```python
from build123d import *

# Parameters (mm, degrees)
F1_DEPTH       = 25.4
F3_D           = 7.874
F3_CBORE_D     = 12.7
F3_CBORE_DEPTH = 6.096
F5_DEPTH       = 12.7
F6_DEPTH       = 105.8292752574
F7_W           = 19.304
F7_H           = 6.096
F8_DEPTH       = 66.549


with BuildPart() as f1:
    # F0 (on Front) → F1 (new body, symmetric)
    with BuildSketch(Plane.XZ):
        Polygon((-85.852, 0), (0, 0), (45.8512699094, -45.8512699094), (54.8315260304, -36.8710137883), (5.2605122421, 12.7), (-85.852, 12.7), align=None)
    extrude(amount=F1_DEPTH, both=True)

    # F3 (through all)
    with Locations(Plane(origin=(0, 0, 0), x_dir=(1, 0, 0), z_dir=(0, 0, -1))):
        with Locations((-70.104, 12.7), (-16.256, 12.7), (-16.256, -12.7), (-70.104, -12.7)):
            CounterBoreHole(F3_D / 2, F3_CBORE_D / 2, F3_CBORE_DEPTH)

    # F4 (on face) → F5 (join)
    with BuildSketch(Plane(origin=(8.9802561211, 0, 8.9802561211), x_dir=(0.7071067812, 0, -0.7071067812), z_dir=(0.7071067812, 0, 0.7071067812))):
        with BuildLine():
            Line((10.9954877579, -25.4), (58.4765061126, -25.4))
            ThreePointArc((58.4765061126, -25.4), (64.8434877579, 0), (58.4765061126, 25.4))
            Line((58.4765061126, 25.4), (10.9954877579, 25.4))
            Line((10.9954877579, 25.4), (10.9954877579, -25.4))
        make_face()
    extrude(amount=F5_DEPTH)

    # F6 (cut, through all): faces of the model
    f6_faces = [f1.faces().sort_by_distance(p)[0] for p in [
        (53.495770348, -19.1275210106, -35.5352581058),
        (53.495770348, 19.1275210106, -35.5352581058),
    ]]
    extrude(f6_faces, amount=-F6_DEPTH, mode=Mode.SUBTRACT)

    # F7 (on face) → F8 (cut, through all)
    with BuildSketch(Plane(origin=(7.774983956, 0, -7.774983956), x_dir=(0, -1, 0), z_dir=(-0.7071067812, 0, 0.7071067812))):
        Polygon((-15.748, 19.304), (-15.748, 12.7), (15.748, 12.7), (15.748, 19.304), (9.652, 19.304), (-9.652, 19.304), align=None)
        with Locations((0, 22.352)):
            Rectangle(F7_W, F7_H)
    extrude(amount=-F8_DEPTH, mode=Mode.SUBTRACT)


solid = f1.part
```
For this review, take the finished solid that the model builds, in its own axes (mm). A direction names the side the tool comes from. Round coordinates to 2 decimals unless told otherwise and drop trailing zeros. Write each loop counter-clockwise with the first axis right and the second up, starting at its lowest first coordinate (ties: lowest second). Pieces come first, ordered by that corner, then holes. Notation, with made-up numbers: (-28, -27.75) - (-9, -27.75) arc R13 cw to (-9, -21.75) - close; hole circle Ø8 at (15.25, 73.25). An arc over 180 degrees is marked (long way). Use CSV: the item, a comma, the result in double quotes.
1) Add section D-D on z = -13.5. Write out the cut boundary in (x, y).
Conclusion:
outline,"(13.5, -25.4) - (49.42, -25.4) - (49.42, -9.65) - (40.8, -9.65) - (40.8, -15.75) - (31.46, -15.75) - (31.46, 15.75) - (40.8, 15.75) - (40.8, 9.65) - (49.42, 9.65) - (49.42, 25.4) - (13.5, 25.4) - close"
2) Add section A-A on y = 12.7. Write out the cut boundary in (x, z) (1 decimal), and give its area (3 significant figures).
Conclusion:
outline,"(-85.9, 0) - (-76.5, 0) - (-76.5, 6.1) - (-74, 6.1) - (-74, 12.7) - (-85.9, 12.7) - close; (-66.2, 6.1) - (-63.8, 6.1) - (-63.8, 0) - (-22.6, 0) - (-22.6, 6.1) - (-20.2, 6.1) - (-20.2, 12.7) - (-66.2, 12.7) - close; (-12.3, 6.1) - (-9.9, 6.1) - (-9.9, 0) - (0, 0) - (44.8, -44.8) - (53.8, -35.8) - (5.3, 12.7) - (-12.3, 12.7) - close; (21.4, 5.9) - (58.4, -31.1) - (62.7, -26.8) - (25.7, 10.2) - close"
area,"2,020 mm^2"
3) The part is to be moulded in two halves that separate along Y. For faces 1 (the cylindrical face through (53, -0.4, -38.7)), 2 (the flat face through (-67, -16, 6.096)), 3 (the cylindrical face through (-19.89, 14.21, 9.44)), 4 (the flat face through (22.18, -19.17, 6.63)), say which applies: pulls with the +Y half, pulls with the -Y half, needs draft (parallel to the pull), parting line crosses it, or undercut.
Conclusion:
face 1,"parting line crosses it"
face 2,"undercut"
face 3,"undercut"
face 4,"needs draft"
4) For faces 5 (the flat face through (23, 0, -23)), 6 (the cylindrical face through (-17.083, -18.996, 3.005)), 7 (the flat face through (42, 9.652, -10)), 8 (the cylindrical face through (-69.251, 16.543, 9.444)), 9 (the flat face through (21.18, 19.39, 5.63)), list the 3-axis set-ups (+Z, -Z, +X, -X, +Y, -Y) from which the entire face can be reached by the end or side of a thin tool; tool diameter is ignored.
Conclusion:
face 5,"-Z, -X, +Y, -Y"
face 6,"-Z"
face 7,"+Z, +X"
face 8,"+Z, -Z"
face 9,"+Z, +Y, -Y"
5) Add section B-B on x = 34. Write out the cut boundary in (y, z), and give its area (3 significant figures).
Conclusion:
outline,"(-25.4, -34) - (25.4, -34) - (25.4, 1.92) - (9.65, 1.92) - (9.65, -6.7) - (15.75, -6.7) - (15.75, -16.04) - (-15.75, -16.04) - (-15.75, -6.7) - (-9.65, -6.7) - (-9.65, 1.92) - (-25.4, 1.92) - close"
area,"1,360 mm^2"
6) Clearance check with flat-ended pins moving along their axes: pin 1 Ø9 at (x, y) = (-70.104, -12.7) entering from -Z; pin 2 Ø16.5 at (x, y) = (-70.104, -12.7) entering from -Z; pin 3 Ø8 at (y, z) = (2, -3) entering from +X; pin 4 Ø12.5 at (x, z) = (50, -8.5) entering from +Y. State where each tip first meets the part, or that it passes through.
Conclusion:
pin 1,"stops at z = 6.1"
pin 2,"stops at z = 0"
pin 3,"stops at x = 24.96"
pin 4,"stops at y = 25.4"
7) Add section C-C on y = 0. Write out the cut boundary in (x, z), and give its area (3 significant figures).
Conclusion:
outline,"(-85.85, 0) - (0, 0) - (45.85, -45.85) - (54.83, -36.87) - (5.26, 12.7) - (-85.85, 12.7) - close"
area,"1,980 mm^2"
8) Wall thickness on line 1 along X through (y, z) = (-12, 4); line 2 along Y through (x, z) = (33, -4); line 3 along X through (y, z) = (12, 9): over which ranges is each line inside the solid? List them lowest first. Write a range as from..to.
Conclusion:
line 1,"x = -85.85..-76.42, -63.79..-22.57, -9.94..13.96, 23.3..31.92"
line 2,"y = -25.4..-9.65, 9.65..25.4"
line 3,"x = -85.85..-73.98, -66.23..-20.13, -12.38..8.96, 24.55..26.92"
